from build123d import *

# Parameters (mm, degrees)
CROQUIS1_W              = 128.409435803
CROQUIS1_H              = 130
CROQUIS1_W_2            = 1200
SALIENTE_EXTRUIR1_DEPTH = 901


with BuildPart() as part:
    # Croquis1 → Saliente-Extruir1 (new body)
    with BuildSketch(Plane.XY):
        with Locations((64.204717902, 975)):
            Rectangle(CROQUIS1_W, CROQUIS1_H)
        Polygon((0, 910), (0, 780), (256.818871606, 780), (256.818871606, 910), (128.409435803, 910), align=None)
        Polygon((0, 780), (0, 650), (387.93663619, 650), (387.93663619, 780), (256.818871606, 780), align=None)
        Polygon((0, 650), (0, 520), (513.637743212, 520), (513.637743212, 650), (387.93663619, 650), align=None)
        Polygon((0, 520), (0, 390), (689.163594473, 390), (689.163594473, 520), (513.637743212, 520), align=None)
        Polygon((0, 390), (0, 260), (858.219540448, 260), (858.219540448, 390), (689.163594473, 390), align=None)
        Polygon((0, 260), (0, 130), (1027.275486423, 130), (1027.275486423, 260), (858.219540448, 260), align=None)
        with Locations((600, 65)):
            Rectangle(CROQUIS1_W_2, CROQUIS1_H)
        Polygon((1200, 0), (0, 0), (0, -130), (1365.387378374, -130), (1365.387378374, 0), align=None)
        Polygon((1365.387378374, -130), (0, -130), (0, -260), (1546.738302238, -260), (1546.738302238, -130), align=None)
    extrude(amount=SALIENTE_EXTRUIR1_DEPTH)


solid = part.part
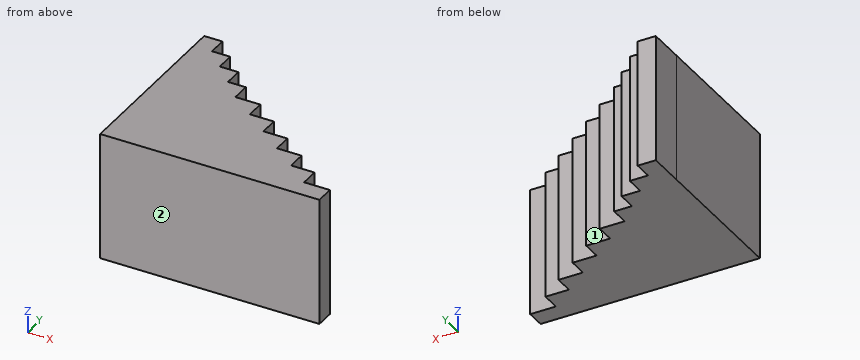
Input: part model. Units: mm. Frame: model coordinates. Face numbers are marked on the shaded views. A direction names the side the tool comes from. Coordinates: 2 decimals unless noted, no trailing zeros. Order: outer loops, then holes, each group sorted by start corner. A loop starts at its lowest first (then second) coordinate and runs counter-clockwise, first axis right, second up. Notation, with made-up numbers: M 11.5,25 L 60.5,25 A28 cw 60.5,49 Z; hole C 71,34.25 d5. An arc over 180 degrees is marked long. One line per question, with ' | ' between items.
Item 1: Pin query (flat end, axial travel): pin 1 (1 mm diameter, centred on y = 216.5, z = 649.5, fed in from +X); pin 2 (4 mm diameter, centred on y = 531, z = 193, fed in from +X). Return the tip coordinate at first contact, or that it passes through.
Geometry results:
pin 1: stops at x = 1027.28 | pin 2: stops at x = 513.64
Item 2: Section C-C (y = 186). Output: boundary loops of the cut face in (x, z).
Geometry results:
outline: M 0,0 L 1027.28,0 L 1027.28,901 L 0,901 Z
Item 3: Reachability of the marked faces 1 and 2 from +Z, -Z, +X, -X, +Y, -Y: full face, straight path, thin tool, end or side. Return the list, or none.
Geometry results:
face 1: +Z, -Z, +X, +Y | face 2: +Z, -Z, +X, -X, -Y
Item 4: Section A-A (z = 593.5). Output: boundary loops of the cut face in (x, y), then the cut area to 3 significant figures.
Geometry results:
outline: M 0,-260 L 1546.74,-260 L 1546.74,-130 L 1365.39,-130 L 1365.39,0 L 1200,0 L 1200,130 L 1027.28,130 L 1027.28,260 L 858.22,260 L 858.22,390 L 689.16,390 L 689.16,520 L 513.64,520 L 513.64,650 L 387.94,650 L 387.94,780 L 256.82,780 L 256.82,910 L 128.41,910 L 128.41,1040 L 0,1040 Z | area: 1,040,000 mm^2
Item 5: Section B-B (x = 286.5). Output: boundary loops of the cut face in (y, z).
Geometry results:
outline: M -260,0 L 780,0 L 780,901 L -260,901 Z
Item 6: Ray query, line 1 along X through (y, z) = (38, 280.5); line 2 along X through (y, z) = (-21, 646); line 3 along Y through (x, z) = (597.5, 364). Return the intervals inside material, ascending.
Geometry results:
line 1: x = 0 to 1200 | line 2: x = 0 to 1365.39 | line 3: y = -260 to 520
